from build123d import *

# Parameters (mm, degrees)
F1_DEPTH = 2025
F2_W     = 10.75
F2_H     = 25
F3_DEPTH = 3.501
F4_W     = 10.75
F4_H     = 3.5
F5_DEPTH = 2000.001


with BuildPart() as f1:
    # F0 (on Top) → F1 (new body)
    with BuildSketch(Plane.XY):
        Polygon((-14.25, 0), (-14.25, -3.5), (10.75, -3.5), (10.75, 0), (0, 0), (0, 25), (-3.5, 25), (-3.5, 0), align=None)
    extrude(amount=F1_DEPTH)

    # F2 (on face) → F3 (cut, through all)
    with BuildSketch(Plane(origin=(0, 0, 0), x_dir=(-1, 0, 0), z_dir=(0, 1, 0))):
        with Locations((8.875, 12.5)):
            Rectangle(F2_W, F2_H)
        Polygon((-10.75, 2012.5), (-10.75, 2000), (0, 2000), (0, 2025), (-10.75, 2025), align=None)
        Polygon((-10.75, 1512.5), (-10.75, 1500), (0, 1500), (0, 1525), (-10.75, 1525), align=None)
        Polygon((-10.75, 1012.5), (-10.75, 1000), (0, 1000), (0, 1025), (-10.75, 1025), align=None)
        Polygon((-10.75, 512.5), (-10.75, 500), (0, 500), (0, 525), (-10.75, 525), align=None)
        Polygon((-10.75, 0), (0, 0), (0, 25), (-10.75, 25), (-10.75, 12.5), align=None)
        with Locations((8.875, 2012.5)):
            Rectangle(F2_W, F2_H)
        with Locations((8.875, 1512.5)):
            Rectangle(F2_W, F2_H)
        with Locations((8.875, 1012.5)):
            Rectangle(F2_W, F2_H)
        with Locations((8.875, 512.5)):
            Rectangle(F2_W, F2_H)
    extrude(amount=-F3_DEPTH, mode=Mode.SUBTRACT)

    # F4 (on face) → F5 (cut, through all)
    with BuildSketch(Plane.XY.offset(2000)):
        with Locations((5.375, -1.75)):
            Rectangle(F4_W, F4_H)
    extrude(amount=-F5_DEPTH, mode=Mode.SUBTRACT)


solid = f1.part
Could you check a few things on this model? Use its own coordinates, in mm. Give positions to 0.01 mm unless a question says otherwise; leave off trailing zeros. Loops run counter-clockwise (first coordinate to the right, second up) from the corner with the lowest first, then second, coordinate; pieces in that order, holes last. Notation, with made-up numbers: M 20,-12.75 L 47,-12.75 A17 ccw 47,8.25 Z; hole C 30.5,-13 d9. An arc over 180 degrees is marked long. Answer as a JSON object with one key per item and string values.
Q1. Suppose I cut it at C-C, the plane y = 8.5. List the corners of the cut face in (x, z) for me, plus the area to 3 significant figures.
Values found:
{"outline": "M -3.5,0 L 0,0 L 0,2025 L -3.5,2025 Z", "area": "7,090 mm²"}
Q2. Suppose I cut it at A-A, the plane x = -6.5. List the corners of the cut face in (y, z) for me.
Values found:
{"outline": "M -3.5,25 L 0,25 L 0,500 L -3.5,500 Z; M -3.5,525 L 0,525 L 0,1000 L -3.5,1000 Z; M -3.5,1025 L 0,1025 L 0,1500 L -3.5,1500 Z; M -3.5,1525 L 0,1525 L 0,2000 L -3.5,2000 Z"}
Q3. Suppose I cut it at B-B, the plane z = 146. List the corners of the cut face in (x, y) for me.
Values found:
{"outline": "M -14.25,-3.5 L 0,-3.5 L 0,25 L -3.5,25 L -3.5,0 L -14.25,0 Z"}
Q4. If I drill on probe 1 along X at (y, z) = (15.75, 743), over which ranges is the centre line in solid material (lowest first)? Write a range as [from, to].
Values found:
{"probe 1": "x = [-3.5, 0]"}
Q5. For P1, Ø4, axis at x = -6.5, y = -1.5, coming from the +Z side; P2, Ø4, axis at x = -6.5, y = -1, coming from the -Z side; P3, Ø5.5, axis at x = -7, z = 1692.5, coming from the +Y side, each with a flat end and sliding along its axis, tell me the tip position at first contact or that it passes through.
Values found:
{"P1": "stops at z = 2000", "P2": "stops at z = 25", "P3": "stops at y = 0"}
